Could you check a few things on this model? Use its own coordinates, in mm. A direction names the side the tool comes from. Give positions to 0.01 mm unless a question says otherwise; leave off trailing zeros. Write each loop counter-clockwise with the first axis right and the second up, starting at its lowest first coordinate (ties: lowest second). Pieces come first, ordered by that corner, then holes. Notation, with made-up numbers: M -34.5,-19.75 L 24.5,-19.75 A14 cw 24.5,-7.75 Z; hole C 42.25,12.5 d5. An arc over 180 degrees is marked long. Answer as a JSON object with one key per item and string values. Group by question number.
```python
from build123d import *

# Parameters (mm, degrees)
SKETCH1_R                    = 60
BOSS_EXTRUDE1_DEPTH          = 70
FILLET2_R                    = 2
SKETCH3_R                    = 55
CUT_EXTRUDE3_DEPTH           = 68
CHAMFER1_SIZE                = 1
BOSS_EXTRUDE3_DEPTH          = 63
FILLET5_R                    = 24.75
M3_CLEARANCE_HOLE1_D         = 3.4
M3_CLEARANCE_HOLE1_DEPTH     = 10
M3_CLEARANCE_HOLE1_TIP       = 1.021463052
M22_CLEARANCE_HOLE1_D        = 20
M18_CLEARANCE_HOLE1_D        = 17.5
SKETCH19_R                   = 1.75
SKETCH19_W                   = 27.8
SKETCH19_H                   = 16
CUT_EXTRUDE4_DEPTH           = 111
CUT_EXTRUDE8_DEPTH           = 111
M2_START                     = 68
M2_CLEARANCE_HOLE1_OUTLINE_R = 1.3
M2_CLEARANCE_HOLE1_DEPTH     = 2


# Read off the part's stored shape, not the designer's step: M2 Clearance Hole1
with BuildPart() as part:
    # Sketch1 → Boss-Extrude1 (new body)
    with BuildSketch(Plane.XY):
        Circle(SKETCH1_R)
    extrude(amount=BOSS_EXTRUDE1_DEPTH)

    # Fillet2
    fillet2_edges = [part.edges().sort_by_distance(p)[0] for p in [
        (-60, 0, 70),
    ]]
    fillet(fillet2_edges, radius=FILLET2_R)

    # Sketch3 → Cut-Extrude3 (cut)
    with BuildSketch(Plane(origin=(0, 0, 0), x_dir=(-1, 0, 0), z_dir=(0, 0, -1))):
        Circle(SKETCH3_R)
    extrude(amount=-CUT_EXTRUDE3_DEPTH, mode=Mode.SUBTRACT)

    # Chamfer1
    chamfer1_edges = [part.edges().sort_by_distance(p)[0] for p in [
        (55, 0, 0),
    ]]
    chamfer(chamfer1_edges, length=CHAMFER1_SIZE)

    # Sketch9 → Boss-Extrude3 (add)
    with BuildSketch(Plane(origin=(0, 0, 5), x_dir=(-1, 0, 0), z_dir=(0, 0, -1))):
        with BuildLine():
            ThreePointArc((-37.067445653, 40.632554347), (-38.890872965, 38.890872965), (-40.632554347, 37.067445653))
            ThreePointArc((-40.632554347, 37.067445653), (-30.757359313, 30.757359313), (-37.067445653, 40.632554347))
        make_face()
        with BuildLine():
            ThreePointArc((-37.067445653, -40.632554347), (-30.757359313, -30.757359313), (-40.632554347, -37.067445653))
            ThreePointArc((-40.632554347, -37.067445653), (-38.890872965, -38.890872965), (-37.067445653, -40.632554347))
        make_face()
        with BuildLine():
            ThreePointArc((37.067445653, 40.632554347), (30.757359313, 30.757359313), (40.632554347, 37.067445653))
            ThreePointArc((40.632554347, 37.067445653), (38.890872965, 38.890872965), (37.067445653, 40.632554347))
        make_face()
        with BuildLine():
            ThreePointArc((40.632554347, -37.067445653), (30.757359313, -30.757359313), (37.067445653, -40.632554347))
            ThreePointArc((37.067445653, -40.632554347), (38.890872965, -38.890872965), (40.632554347, -37.067445653))
        make_face()
    extrude(amount=-BOSS_EXTRUDE3_DEPTH)

    # Fillet5
    fillet5_edges = [part.edges().sort_by_distance(p)[0] for p in [
        (37.067445653, -40.632554347, 36.5),
        (40.632554347, -37.067445653, 36.5),
        (-37.067445653, 40.632554347, 36.5),
        (-40.632554347, 37.067445653, 36.5),
        (-40.632554347, -37.067445653, 36.5),
        (-37.067445653, -40.632554347, 36.5),
        (37.067445653, 40.632554347, 36.5),
        (40.632554347, 37.067445653, 36.5),
    ]]
    fillet(fillet5_edges, radius=FILLET5_R)

    # M3 Clearance Hole1
    with Locations(Plane(origin=(0, 0, 5), x_dir=(-1, 0, 0), z_dir=(0, 0, -1))):
        with Locations((-35, -35), (0, 0), (-35, 35), (35, -35), (35, 35)):
            Hole(M3_CLEARANCE_HOLE1_D / 2, depth=M3_CLEARANCE_HOLE1_DEPTH)
            with Locations((0, 0, -(M3_CLEARANCE_HOLE1_DEPTH + M3_CLEARANCE_HOLE1_TIP / 2))):  # 118° drill point
                Cone(0, M3_CLEARANCE_HOLE1_D / 2, M3_CLEARANCE_HOLE1_TIP, mode=Mode.SUBTRACT)

    # M22 Clearance Hole1 (through all)
    with Locations(Plane.XY.offset(70)):
        with Locations((38.1, 0)):
            Hole(M22_CLEARANCE_HOLE1_D / 2)

    # M18 Clearance Hole1 (through all)
    with Locations(Plane.XY.offset(70)):
        with Locations((-38.1, 0)):
            Hole(M18_CLEARANCE_HOLE1_D / 2)

    # Sketch19 → Cut-Extrude4 (cut, through all)
    with BuildSketch(Plane.XY.offset(70)):
        with Locations((-11.685971223, 11.9)):
            Circle(SKETCH19_R)
        with Locations((11.685971223, 11.9)):
            Circle(SKETCH19_R)
        with Locations((11.685971223, -11.9)):
            Circle(SKETCH19_R)
        with Locations((-11.685971223, -11.9)):
            Circle(SKETCH19_R)
        Rectangle(SKETCH19_W, SKETCH19_H)
    extrude(amount=-CUT_EXTRUDE4_DEPTH, mode=Mode.SUBTRACT)

    # Sketch25 → Cut-Extrude8 (cut, through all)
    with BuildSketch(Plane.XY.offset(70)):
        with BuildLine():
            Line((-4.25, -35.1), (4.25, -35.1))
            ThreePointArc((4.25, -35.1), (7.25, -38.1), (4.25, -41.1))
            Line((4.25, -41.1), (-4.25, -41.1))
            ThreePointArc((-4.25, -41.1), (-7.25, -38.1), (-4.25, -35.1))
        make_face()
    extrude(amount=-CUT_EXTRUDE8_DEPTH, mode=Mode.SUBTRACT)

    # M2 Clearance Hole1 outline → M2 Clearance Hole1 (cut)
    with BuildSketch(Plane.XY.offset(M2_START)):
        with Locations((-9.5, 38.1)):
            Circle(M2_CLEARANCE_HOLE1_OUTLINE_R)
        with Locations((9.5, 38.1)):
            Circle(M2_CLEARANCE_HOLE1_OUTLINE_R)
    extrude(amount=M2_CLEARANCE_HOLE1_DEPTH, mode=Mode.SUBTRACT)


solid = part.part
```
1) If we section it at B-B, the plane y = 0: List the corners of the cut face in (x, z) for me, plus the area to 3 significant figures.
2) If we section it at A-A, the plane x = 0: List the corners of the cut face in (y, z) for me, plus the area to 3 significant figures.
3) Please list where these lines run through material, in increasing order: line 1 along Y through (x, z) = (35, 11); line 2 along Z through (x, y) = (7, 34.5); line 3 along Y through (x, z) = (44, 4.5). Write a range as from..to.
4) For faces 1 (the cylindrical face through (30.794, 30.721, 36.059)), 2 (the cylindrical face through (-7.25, -38.17, 69.01)), which set-ups out of +Z, -Z, +X, -X, +Y, -Y let a thin tool reach every point of the face, with its end or its side?
5) I'm going to push flat-ended pins straight in: pin 1 (3 mm diameter, centred on y = -35, z = 26.5, fed in from +X); pin 2 (4 mm diameter, centred on x = 32.5, z = 52.5, fed in from +Y); pin 3 (2 mm diameter, centred on x = 11.69, y = 11.9, fed in from -Z); pin 4 (3 mm diameter, centred on x = 34, z = 10, fed in from -Y). Where does each tip first touch, or does it pass through?
6) We'd pull the mould along X, two halves only. Please class faces 3 (the flat face through (40, -40, 0)), 4 (the conical face through (34.718, -34.911, 15.844)), 5 (the cylindrical face through (-59.94, 2.64, 33.52)): released by +X, released by -X, zero draft, split by the parting line, or undercut.
Taken from the geometry:
{
 "1": {"outline": "M -60,0 L -56,0 L -55,1 L -55,68 L -46.85,68 L -46.85,70 L -58,70 A2 ccw -60,68 Z; M -29.35,68 L -13.9,68 L -13.9,70 L -29.35,70 Z; M 13.9,68 L 28.1,68 L 28.1,70 L 13.9,70 Z; M 48.1,68 L 55,68 L 55,1 L 56,0 L 60,0 L 60,68 A2 ccw 58,70 L 48.1,70 Z", "area": "787 mm²"},
 "2": {"outline": "M -60,0 L -56,0 L -55,1 L -55,68 L -41.1,68 L -41.1,70 L -58,70 A2 ccw -60,68 Z; M -35.1,68 L -8,68 L -8,70 L -35.1,70 Z; M 8,68 L 55,68 L 55,1 L 56,0 L 60,0 L 60,68 A2 ccw 58,70 L 8,70 Z", "area": "873 mm²"},
 "3": {"line 1": "-48.73..-36.7, -33.3..-28.89, 28.89..33.3, 36.7..48.73", "line 2": "68..70", "line 3": "-40.79..-33, 33..40.79"},
 "4": {"face 1": "-Z", "face 2": "+Z, -Z"},
 "5": {"pin 1": "x = 49.78", "pin 2": "y = 51.67", "pin 3": "through", "pin 4": "y = -50.44"},
 "6": {"face 3": "zero draft", "face 4": "undercut", "face 5": "split by the parting line"}
}
